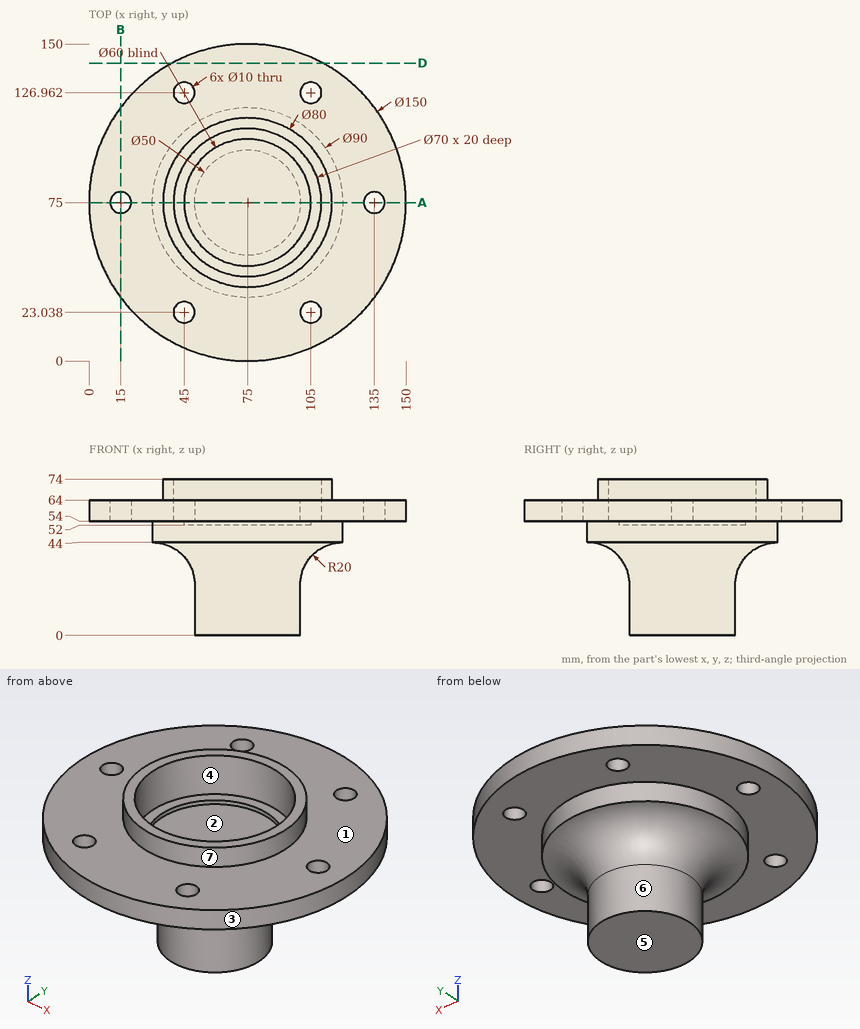
The figure shows three views and two pictorial views of one solid part (mm, origin at its lowest corner). Answer the questions. A direction names the side the tool comes from. Round coordinates to 2 decimals unless told otherwise and drop trailing zeros. Loops run counter-clockwise (first coordinate to the right, second up) from the corner with the lowest first, then second, coordinate; pieces in that order, holes last. Notation, with made-up numbers: M -17,36 L 30,36 A7 cw 30,44 Z; hole C 37,-17.5 d7. An arc over 180 degrees is marked long. Write each question's results on one line, items separated by ' | '. Start each with the question number.
1) Straight lines are drawn through the part: probe 1 along Y at (x, z) = (135, 57); probe 2 along Y at (x, z) = (105, 57.75) (1 decimal); probe 3 along Y at (x, z) = (75, 65). For each, find the intervals that lie inside material, in ascending order.
2) Determine the mould class of the marked faces 1, 2, 3 and 4 for opening direction X: pulls with the +X half, pulls with the -X half, needs draft (parallel to the pull), parting line crosses it, or undercut.
3) Find section D-D on y = 141. Write down the section's boundary in (x, z).
4) Find section B-B on x = 15. Write down the section's boundary in (y, z), plus the area to 3 significant figures.
5) Each of these flat-tipped pins is pushed along its axis until it touches: pin 1 (6 mm diameter, centred on x = 16.5, z = 62.5, fed in from -Y) (1 decimal); pin 2 (4 mm diameter, centred on x = 108.5, y = 124, fed in from -Z); pin 3 (1 mm diameter, centred on x = 91.5, y = 76, fed in from +Z). Where does it stop, or does it pass through?
6) Which of the six approach directions +Z, -Z, +X, -X, +Y, -Y give full straight-line access (tool end or side, diameter ignored) to the marked faces 5, 6 and 7?
7) Find section A-A on y = 75. Count the separate pieces of the cut face and the enclosed holes in it, plus the area to 3 significant figures.
Final values:
1) probe 1: 30 to 70, 80 to 120 | probe 2: 6.3 to 18, 28 to 57, 93 to 122, 132 to 143.7 | probe 3: 35 to 40, 110 to 115
2) face 1: needs draft | face 2: undercut | face 3: parting line crosses it | face 4: undercut
3) outline: M 39.38,54 L 110.62,54 L 110.62,64 L 39.38,64 Z
4) outline: M 30,54 L 70,54 L 70,64 L 30,64 Z; M 80,54 L 120,54 L 120,64 L 80,64 Z | area: 800 mm²
5) pin 1: y = 24.6 | pin 2: z = 54 | pin 3: z = 52
6) face 5: -Z, +X, -X, +Y, -Y | face 6: -Z | face 7: +Z
7) separate pieces: 3 | enclosed holes: 0 | area: 3,850 mm²
